Check sheet for the modelled part. Datum: model origin and axes. Units: mm. A direction names the side the tool comes from. Give positions to 0.01 mm unless a question says otherwise; leave off trailing zeros. Order: outer loops, then holes, each group sorted by start corner. A loop starts at its lowest first (then second) coordinate and runs counter-clockwise, first axis right, second up. Notation, with made-up numbers: M 49,79.5 L 60,79.5 A29 cw 60,112.5 Z; hole C -27,16 d5. An arc over 180 degrees is marked long. Answer in a Markdown table with one row per item. Add a question column.
from build123d import *

# Parameters (mm, degrees)
SKETCH1_R           = 2.25
SKETCH1_R_2         = 1.65
SKETCH1_R_3         = 1.25282433
SKETCH1_W           = 40.6
SKETCH1_H           = 20.8
BOSS_EXTRUDE1_DEPTH = 3.175


with BuildPart() as part:
    # Sketch1 → Boss-Extrude1 (new body)
    with BuildSketch(Plane(origin=(0, 0, 0), x_dir=(1, 0, 0), z_dir=(0, 1, 0))):
        with BuildLine():
            Line((-162.38735588, 17.244652891), (-102.38735588, 17.244652891))
            Line((-102.38735588, 17.244652891), (7.61264412, 12.244652891))
            ThreePointArc((7.61264412, 12.244652891), (17.61264412, 2.244652891), (7.61264412, -7.755347109))
            Line((7.61264412, -7.755347109), (-102.38735588, -12.755347109))
            Line((-102.38735588, -12.755347109), (-162.38735588, -12.755347109))
            ThreePointArc((-162.38735588, -12.755347109), (-177.38735588, 2.244652891), (-162.38735588, 17.244652891))
        make_face()
        with Locations(Location((-168.38735588, 7.244652891, 0), (0, 0, 270))):
            Circle(SKETCH1_R, mode=Mode.SUBTRACT)
        with Locations(Location((-168.38735588, -2.755347109, 0), (0, 0, 270))):
            Circle(SKETCH1_R, mode=Mode.SUBTRACT)
        with Locations(Location((-118.78735588, 7.244652891, 0), (0, 0, 270))):
            Circle(SKETCH1_R, mode=Mode.SUBTRACT)
        with Locations(Location((-118.78735588, -2.755347109, 0), (0, 0, 270))):
            Circle(SKETCH1_R, mode=Mode.SUBTRACT)
        with Locations(Location((-42.38735588, 2.244652891, 0), (0, 0, 270))):
            Circle(SKETCH1_R_2, mode=Mode.SUBTRACT)
        with Locations(Location((3.23764412, 2.246310682, 0), (0, 0, 270))):
            Circle(SKETCH1_R_3, mode=Mode.SUBTRACT)
        with Locations((-142.392621679, 2.244652891)):
            Rectangle(SKETCH1_W, SKETCH1_H, mode=Mode.SUBTRACT)
    extrude(amount=BOSS_EXTRUDE1_DEPTH)


solid = part.part
Q1. Thickness scan on probe 1 along Z at (x, y) = (-145, 2); probe 2 along X at (y, z) = (1.4, -1.5); probe 3 along Z at (x, y) = (-102, 0.35). Record the ranges inside material, lowest first.
Q2. Tool access check on faces 1 (the flat face through (-162.693, 2, -2)), 2 (the cylindrical face through (17.61, 1.57, -2.46)). Record the directions out of +Z, -Z, +X, -X, +Y, -Y that give a thin tool (end or side, any length) a straight path to the whole face; none if there is none.
Q3. Cross-section at D-D (z = 3). Record the boundary of the cut face in (x, y) (3 decimals), and give its area (3 significant figures).
Q4. Cross-section at C-C (y = 2.05). Record the boundary of the cut face in (x, z).
Q5. Go/stop test with flat-tipped pins: pin 1 (2 mm diameter, centred on x = -42.39, z = -2.24, fed in from +Y); pin 2 (1 mm diameter, centred on y = 1.5, z = -4, fed in from +X). Record where each tip stops, or that it passes through.
Q6. Cross-section at B-B (z = -7.5). Record the boundary of the cut face in (x, y) (3 decimals), and give its area (3 significant figures).
Q7. Draft check along Z on faces 3 (the cylindrical face through (-116.557, 1.565, -7.538)), 4 (the flat face through (-132, 2, 12.755)), 5 (the flat face through (-79, 3.175, -2)), 6 (the cylindrical face through (-116.557, 1.565, 2.462)). Enter one of: pulls with the +Z half, pulls with the -Z half, needs draft (parallel to the pull), parting line crosses it, or undercut.
Q8. Cross-section at A-A (x = -127). Record the boundary of the cut face in (y, z) (3 decimals).
Values follow:
| question | item | result |
|---|---|---|
| 1 | probe 1 | -17.24 to -12.64, 8.16 to 12.76 |
| 1 | probe 2 | -177.37 to -162.69, -122.09 to -43.86, -40.91 to 2.23, 4.24 to 17.58 |
| 1 | probe 3 | -17.23 to 12.74 |
| 2 | face 1 | +Y, -Y |
| 2 | face 2 | +X, +Y, -Y |
| 3 | outline | M -176.441,0 L -170.624,0 L -170.624,3.175 L -176.441,3.175 Z; M -166.151,0 L -162.693,0 L -162.693,3.175 L -166.151,3.175 Z; M -122.093,0 L -121.024,0 L -121.024,3.175 L -122.093,3.175 Z; M -116.551,0 L 16.127,0 L 16.127,3.175 L -116.551,3.175 Z |
| 3 | area | 454 mm² |
| 4 | outline | M -162.39,-17.24 L -102.39,-17.24 L 7.61,-12.24 A10 ccw 7.61,7.76 L -102.39,12.76 L -162.39,12.76 A15 ccw Z; hole C -168.39,-7.24 d4.5; hole C -168.39,2.76 d4.5; hole M -162.69,-12.64 L -122.09,-12.64 L -122.09,8.16 L -162.69,8.16 Z; hole C -118.79,-7.24 d4.5; hole C -118.79,2.76 d4.5; hole C -42.39,-2.24 d3.3; hole C 3.24,-2.25 d2.51 |
| 5 | pin 1 | through |
| 5 | pin 2 | x = 17.53 |
| 6 | outline | M -176.437,0 L -170.623,0 L -170.623,3.175 L -176.437,3.175 Z; M -166.152,0 L -162.693,0 L -162.693,3.175 L -166.152,3.175 Z; M -122.093,0 L -121.023,0 L -121.023,3.175 L -122.093,3.175 Z; M -116.552,0 L 16.12,0 L 16.12,3.175 L -116.552,3.175 Z |
| 6 | area | 454 mm² |
| 7 | face 3 | undercut |
| 7 | face 4 | pulls with the +Z half |
| 7 | face 5 | needs draft |
| 7 | face 6 | undercut |
| 8 | outline | M 0,-17.245 L 3.175,-17.245 L 3.175,-12.645 L 0,-12.645 Z; M 0,8.155 L 3.175,8.155 L 3.175,12.755 L 0,12.755 Z |
